The model under review builds one solid part; all positions refer to its coordinate system, in mm. A direction names the side the tool comes from. Round coordinates to 2 decimals unless told otherwise and drop trailing zeros. Loops run counter-clockwise (first coordinate to the right, second up) from the corner with the lowest first, then second, coordinate; pieces in that order, holes last. Notation, with made-up numbers: (66.5, 36.5) -> (91.5, 36.5) arc R9 cw to (91.5, 42.5) -> close; hole circle Ø11 at (-2, -34.5). An arc over 180 degrees is marked (long way). Use a Markdown table: item, result. Add a question column.
1) Consider section D-D on z = -24. Give the boundary of the cut face in (x, y), plus the area to 3 significant figures.
2) Consider section A-A on x = 11. Give the boundary of the cut face in (y, z), plus the area to 3 significant figures.
3) Consider section B-B on z = -29. Give the boundary of the cut face in (x, y), plus the area to 3 significant figures.
4) Mouldability with a two-part tool opening along X and no side actions: class faces 1 (the flat face through (35, 4, -11)), 2 (the flat face through (17, 8, -18)), 3 (the cylindrical face through (22.5, 3.94, -10.93)), 4 (the cylindrical face through (25.8, 2, -8.4)) as released by +X, released by -X, zero draft, split by the parting line, or undercut.
5) For faces 5 (the flat face through (2, 4, -17)), 6 (the flat face through (13, 4, -30)), 7 (the flat face through (8.5, -40, -17)), list the 3-axis set-ups (+Z, -Z, +X, -X, +Y, -Y) from which the entire face can be reached by the end or side of a thin tool; tool diameter is ignored.
6) Wall thickness on probe 1 along Z at (x, y) = (24, 5.25); probe 2 along Z at (x, y) = (11, 4); probe 3 along Z at (x, y) = (6, 2.95): over which ranges is each line inside the solid? List them lowest first.
7) Consider section C-C on y = -3. Give the boundary of the cut face in (x, z), plus the area to 3 significant figures.
8) Insertion check: pin 1 (5.5 mm diameter, centred on x = 21.5, y = 3, fed in from +Z); pin 2 (1.5 mm diameter, centred on y = 4, z = -2.5, fed in from +X); pin 3 (3 mm diameter, centred on y = -21.5, z = -19, fed in from -X); pin 4 (6.5 mm diameter, centred on x = 27.5, z = -6, fed in from -Y). Each pin has a flat end and moves straight along its axis. Give the tip position at first contact, or say it passes through.
from build123d import *

# Parameters (mm, degrees)
SKETCH1_W           = 35
SKETCH1_H           = 35
BOSS_EXTRUDE1_DEPTH = 8
SKETCH2_W           = 5
SKETCH2_H           = 7
SKETCH2_W_2         = 7
SKETCH2_H_2         = 5
SKETCH2_R           = 1.5
CUT_EXTRUDE1_DEPTH  = 9
SKETCH2_5_R         = 4
SKETCH2_5_R_2       = 1.5
CUT_EXTRUDE2_DEPTH  = 4
SKETCH2_7_R         = 5
SKETCH2_7_R_2       = 2.5
BOSS_EXTRUDE2_DEPTH = 38.25
SKETCH3_W           = 18
SKETCH3_H           = 18
BOSS_EXTRUDE3_DEPTH = 4
FILLET1_R           = 5


with BuildPart() as part:
    # Sketch1 → Boss-Extrude1 (new body)
    with BuildSketch(Plane(origin=(0, 0, 0), x_dir=(1, 0, 0), z_dir=(0, 1, 0))):
        with Locations((17.5, 17.5)):
            Rectangle(SKETCH1_W, SKETCH1_H)
    extrude(amount=BOSS_EXTRUDE1_DEPTH)

    # Sketch2 → Cut-Extrude1 (cut, through all)
    with BuildSketch(Plane.XZ):
        with Locations((32.5, -21.5)):
            Rectangle(SKETCH2_W, SKETCH2_H)
        with Locations((13.5, -32.5)):
            Rectangle(SKETCH2_W_2, SKETCH2_H_2)
        with Locations((2.5, -13.5)):
            Rectangle(SKETCH2_W, SKETCH2_H)
        with Locations((21.5, -2.5)):
            Rectangle(SKETCH2_W_2, SKETCH2_H_2)
        with Locations((11, -11)):
            Circle(SKETCH2_R)
        with Locations((24, -11)):
            Circle(SKETCH2_R)
        with Locations((11, -24)):
            Circle(SKETCH2_R)
        with Locations((24, -24)):
            Circle(SKETCH2_R)
    extrude(amount=-CUT_EXTRUDE1_DEPTH, mode=Mode.SUBTRACT)

    # Sketch2_5 → Cut-Extrude2 (cut)
    with BuildSketch(Plane.XZ):
        with Locations((6, -29)):
            Circle(SKETCH2_5_R)
        with Locations((29, -6)):
            Circle(SKETCH2_5_R)
        with Locations((11, -11)):
            Circle(SKETCH2_5_R_2)
    extrude(amount=-CUT_EXTRUDE2_DEPTH, mode=Mode.SUBTRACT)

    # Sketch2_7 → Boss-Extrude2 (add)
    with BuildSketch(Plane.XZ):
        with Locations((17.5, -17.5)):
            Circle(SKETCH2_7_R)
        with Locations((29, -29)):
            Circle(SKETCH2_7_R_2)
        with Locations((6, -6)):
            Circle(SKETCH2_7_R_2)
    extrude(amount=BOSS_EXTRUDE2_DEPTH)

    # Sketch3 → Boss-Extrude3 (add)
    with BuildSketch(Plane(origin=(0, -38.25, 0), x_dir=(-1, 0, 0), z_dir=(0, -1, 0))):
        with Locations((-17.5, 17.5)):
            Rectangle(SKETCH3_W, SKETCH3_H)
    extrude(amount=BOSS_EXTRUDE3_DEPTH)

    # Fillet1
    fillet1_edges = [part.edges().sort_by_distance(p)[0] for p in [
        (0, 4, -35),
        (35, 4, -35),
        (35, 4, 0),
        (0, 4, 0),
    ]]
    fillet(fillet1_edges, radius=FILLET1_R)


solid = part.part
Result set:
| question | item | result |
|---|---|---|
| 1 | outline | (0, 0) -> (9.5, 0) -> (9.5, 8) -> (0, 8) -> close; (8.5, -42.25) -> (26.5, -42.25) -> (26.5, -38.25) -> (8.5, -38.25) -> close; (12.5, 0) -> (22.5, 0) -> (22.5, 8) -> (12.5, 8) -> close; (25.5, 0) -> (30, 0) -> (30, 8) -> (25.5, 8) -> close |
| 1 | area | 264 mm2 |
| 2 | outline | (-42.25, -26.5) -> (-38.25, -26.5) -> (-38.25, -8.5) -> (-42.25, -8.5) -> close; (0, -30) -> (8, -30) -> (8, -25.5) -> (0, -25.5) -> close; (0, -22.5) -> (8, -22.5) -> (8, -12.5) -> (0, -12.5) -> close; (0, -9.5) -> (8, -9.5) -> (8, 0) -> (0, 0) -> close |
| 2 | area | 264 mm2 |
| 3 | outline | (0, 0) -> (2, 0) -> (2, 4) -> (10, 4) -> (10, 0) -> (26.5, 0) -> (26.5, -38.25) -> (31.5, -38.25) -> (31.5, 0) -> (35, 0) -> (35, 8) -> (0, 8) -> close |
| 3 | area | 439 mm2 |
| 4 | face 1 | released by +X |
| 4 | face 2 | zero draft |
| 4 | face 3 | undercut |
| 4 | face 4 | undercut |
| 5 | face 5 | -X, +Y, -Y |
| 5 | face 6 | -Z, +Y, -Y |
| 5 | face 7 | +Z, -Z, -X, -Y |
| 6 | probe 1 | -35 to -25.5, -22.5 to -12.5, -9.5 to -5 |
| 6 | probe 2 | -30 to -25.5, -22.5 to -12.5, -9.5 to 0 |
| 6 | probe 3 | -35 to -33, -25 to 0 |
| 7 | outline | circle Ø5 at (6, -6); circle Ø10 at (17.5, -17.5); circle Ø5 at (29, -29) |
| 7 | area | 118 mm2 |
| 8 | pin 1 | z = -5 |
| 8 | pin 2 | x = 34.68 |
| 8 | pin 3 | x = 12.5 |
| 8 | pin 4 | y = -42.25 |
